from build123d import *

# Parameters (mm, degrees)
SKETCH1_W           = 38.1
SKETCH1_H           = 50.8
BOSS_EXTRUDE1_DEPTH = 6.35
SKETCH2_R           = 2.15265
CUT_EXTRUDE1_DEPTH  = 25.4


with BuildPart() as part:
    # Sketch1 → Boss-Extrude1 (new body)
    with BuildSketch(Plane(origin=(0, 0, 0), x_dir=(1, 0, 0), z_dir=(0, 1, 0))):
        Rectangle(SKETCH1_W, SKETCH1_H)
    extrude(amount=BOSS_EXTRUDE1_DEPTH)

    # Sketch2 → Cut-Extrude1 (cut)
    with BuildSketch(Plane.ZY.offset(19.05)):
        with Locations((-19.05, 3.175)):
            Circle(SKETCH2_R)
        with Locations((0, 3.175)):
            Circle(SKETCH2_R)
        with Locations((19.05, 3.175)):
            Circle(SKETCH2_R)
    cut_extrude1 = extrude(amount=-CUT_EXTRUDE1_DEPTH, mode=Mode.SUBTRACT)

    # Mirror1: Cut-Extrude1 across plane
    add(cut_extrude1.mirror(Plane(origin=(0, 0, 0), x_dir=(0, 0, 1), z_dir=(1, 0, 0))), mode=Mode.SUBTRACT)


solid = part.part
Build history of the part. All positions in model axes, mm. Give positions to 0.01 mm unless a question says otherwise; leave off trailing zeros. Order: outer loops, then holes, each group sorted by start corner. A loop starts at its lowest first (then second) coordinate and runs counter-clockwise, first axis right, second up. Notation, with made-up numbers: M -12,29 L 11,29 A10 cw 11,36 Z; hole C 39,-38.75 d2. An arc over 180 degrees is marked long. Put each result on its own line as item: value.
Item 1: Cut at C-C on y = 4.25. Write the cut outline in (x, z).
Results are:
outline: M -19.05,-25.4 L 19.05,-25.4 L 19.05,-20.92 L -19.05,-20.92 Z; M -19.05,-17.18 L 19.05,-17.18 L 19.05,-1.87 L -19.05,-1.87 Z; M -19.05,1.87 L 19.05,1.87 L 19.05,17.18 L -19.05,17.18 Z; M -19.05,20.92 L 19.05,20.92 L 19.05,25.4 L -19.05,25.4 Z
Item 2: Cut at A-A on z = 0. Write the cut outline in (x, y).
Results are:
outline: M -19.05,0 L 19.05,0 L 19.05,1.02 L -19.05,1.02 Z; M -19.05,5.33 L 19.05,5.33 L 19.05,6.35 L -19.05,6.35 Z
Item 3: Cut at D-D on z = 19.5. Write the cut outline in (x, y).
Results are:
outline: M -19.05,0 L 19.05,0 L 19.05,1.07 L -19.05,1.07 Z; M -19.05,5.28 L 19.05,5.28 L 19.05,6.35 L -19.05,6.35 Z
Item 4: Drop a flat-ended pin along its axis: pin 1 Ø3.5 at (y, z) = (3.175, 19.05) entering from +X. Give the stop position or say it passes through.
Results are:
pin 1: through
Item 5: Wall check: probe 1 along Y at (x, z) = (-1, 0); probe 2 along Z at (x, y) = (9, 1.75); probe 3 along Z at (x, y) = (12.5, 2). Give the ranges that are in metal, low to high.
Results are:
probe 1: 0 to 1.02, 5.33 to 6.35
probe 2: -25.4 to -20.66, -17.44 to -1.61, 1.61 to 17.44, 20.66 to 25.4
probe 3: -25.4 to -20.85, -17.25 to -1.8, 1.8 to 17.25, 20.85 to 25.4
Item 6: Cut at B-B on x = 16. Write the cut outline in (y, z) (3 decimals).
Results are:
outline: M 0,-25.4 L 6.35,-25.4 L 6.35,25.4 L 0,25.4 Z; hole C 3.175,-19.05 d4.305; hole C 3.175,0 d4.305; hole C 3.175,19.05 d4.305
